Part model, mm, in its own coordinate system. Give positions to 0.01 mm unless a question says otherwise; leave off trailing zeros. Write each loop counter-clockwise with the first axis right and the second up, starting at its lowest first coordinate (ties: lowest second). Pieces come first, ordered by that corner, then holes.
```python
from build123d import *


with BuildPart() as part:
    # Sketch1 → Revolve1 (revolve)
    with BuildSketch(Plane(origin=(0, 0, 0), x_dir=(0, 0, -1), z_dir=(1, 0, 0)), mode=Mode.PRIVATE) as revolve1_sk:
        Polygon((-197, 0), (153, 0), (153, 4), (150.9, 4), (150.9, 3.8), (150, 3.8), (150, 4), (143, 4), (143, 6), (-143, 6), (-143, 5), (-166, 5), (-166, 4), (-168, 4), (-168, 5), (-182, 5), (-182, 4), (-197, 4), align=None)
    revolve(revolve1_sk.sketch.rotate(Axis((0, 0, 197), (0, 0, -1)), 90), axis=Axis((0, 0, 197), (0, 0, -1)))


solid = part.part
```
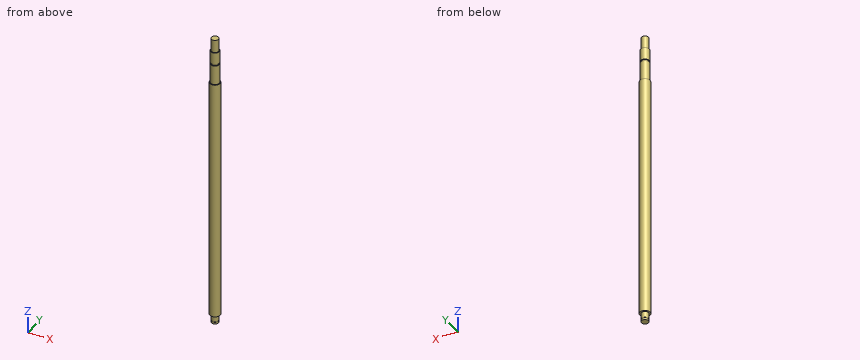
1) Saw through at D-D, the plane z = 163. Write the cut outline in (x, y).
Answers follow:
outline: circle Ø10 at (0, 0)
2) Saw through at C-C, the plane z = -130. Write the cut outline in (x, y), then the cut area to 3 significant figures.
Answers follow:
outline: circle Ø12 at (0, 0)
area: 113 mm2
3) Pin check, flat tips, straight feed: pin 1 Ø1 at (y, z) = (1, -108) entering from -X; pin 2 Ø1.5 at (y, z) = (-2, -81.5) entering from -X; pin 3 Ø2 at (y, z) = (-4, 45.5) entering from +X. Stop position of each tip, or through.
Answers follow:
pin 1: stops at x = -5.98
pin 2: stops at x = -5.87
pin 3: stops at x = 5.2
4) Wall check: L1, parallel to Z at x = -4, y = 0.5; L2, parallel to Z at x = 3.75, y = -1; L3, parallel to X at y = -4.5, z = -100.5. Give the ranges that are in metal, low to high.
Answers follow:
L1: z = -143 to 166, 168 to 182
L2: z = -153 to -150.9, -150 to 197
L3: x = -3.97 to 3.97
